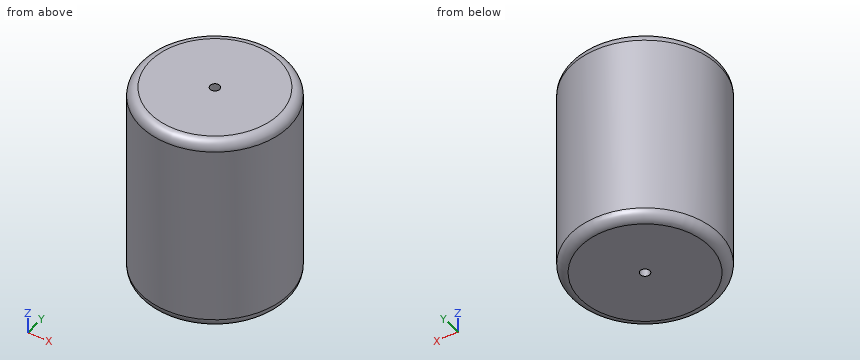
```python
from build123d import *

# Parameters (mm, degrees)
SKETCH1_R           = 7.75
BOSS_EXTRUDE1_DEPTH = 21
FILLET1_R           = 1
SKETCH2_R           = 0.505
CUT_EXTRUDE1_DEPTH  = 51.7


with BuildPart() as part:
    # Sketch1 → Boss-Extrude1 (new body)
    with BuildSketch(Plane.XY):
        Circle(SKETCH1_R)
    extrude(amount=BOSS_EXTRUDE1_DEPTH)

    # Fillet1
    fillet1_edges = [part.edges().sort_by_distance(p)[0] for p in [
        (-7.75, 0, 0),
        (-7.75, 0, 21),
    ]]
    fillet(fillet1_edges, radius=FILLET1_R)

    # Sketch2 → Cut-Extrude1 (cut)
    with BuildSketch(Plane.XY.offset(21)):
        Circle(SKETCH2_R)
    extrude(amount=-CUT_EXTRUDE1_DEPTH, mode=Mode.SUBTRACT)


solid = part.part
```
Input: part model. Units: mm. Frame: model coordinates. Coordinates: 2 decimals unless noted, no trailing zeros. Loops run counter-clockwise (first coordinate to the right, second up) from the corner with the lowest first, then second, coordinate; pieces in that order, holes last. Notation, with made-up numbers: M -13,70.5 L -8,70.5 A12 ccw -8,87.5 Z; hole C -29,-12.75 d8. An arc over 180 degrees is marked long. Use a Markdown table: item, result. Add a question column.
1) Section A-A, the plane x = 0. Return the cut outline in (y, z) (3 decimals), plus the area to 3 significant figures.
2) Line query: L1, parallel to Y at x = 0, z = 13.5 (3 decimals); L2, parallel to X at y = 0.25, z = 4.25; L3, parallel to Y at x = -5.5, z = 1.75. Output: solid intervals per line, ascending. Write a range as from..to.
3) Section C-C, the plane z = 5. Return the cut outline in (x, y) (3 decimals), plus the area to 3 significant figures.
4) Pin query (flat end, axial travel): P1, Ø6, axis at y = 2, z = 17, coming from the +X side; P2, Ø5, axis at x = 5.5, z = 12, coming from the -Y side; P3, Ø3, axis at y = -4, z = 18.5, coming from the -X side; P4, Ø3, axis at y = 3, z = 13.5, coming from the -X side. Return the tip coordinate at first contact, or that it passes through.
Answer below:
| question | item | result |
|---|---|---|
| 1 | outline | M -7.75,1 A1 ccw -6.75,0 L -0.505,0 L -0.505,21 L -6.75,21 A1 ccw -7.75,20 Z; M 0.505,0 L 6.75,0 A1 ccw 7.75,1 L 7.75,20 A1 ccw 6.75,21 L 0.505,21 Z |
| 1 | area | 303 mm2 |
| 2 | L1 | -7.75..-0.505, 0.505..7.75 |
| 2 | L2 | -7.75..-0.44, 0.44..7.75 |
| 2 | L3 | -5.46..5.46 |
| 3 | outline | C 0,0 d15.5; hole C 0,0 d1.01 |
| 3 | area | 188 mm2 |
| 4 | P1 | x = 7.75 |
| 4 | P2 | y = -7.15 |
| 4 | P3 | x = -7.34 |
| 4 | P4 | x = -7.6 |
